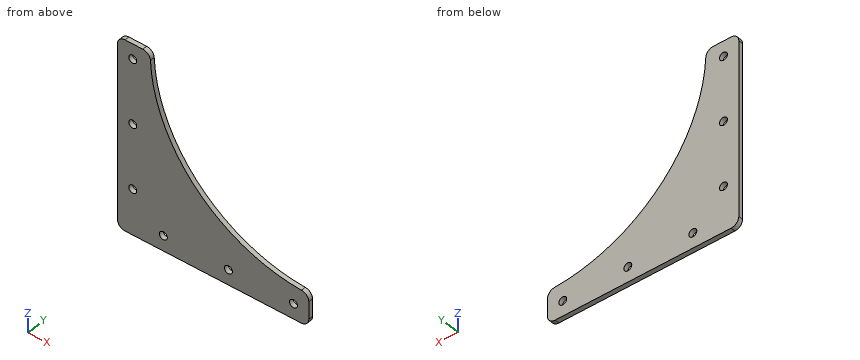
from build123d import *

# Parameters (mm, degrees)
F0_R     = 2.6
F1_DEPTH = 3


with BuildPart() as f1:
    # F0 (on Front) → F1 (new body)
    with BuildSketch(Plane.XZ):
        with BuildLine():
            Line((-57.5, -62.5), (57.5, -62.5))
            ThreePointArc((57.5, -62.5), (61.035534, -61.035534), (62.5, -57.5))
            Line((62.5, -57.5), (62.5, -45.930671))
            ThreePointArc((62.5, -45.930671), (61.116047, -42.477526), (57.730317, -40.935978))
            ThreePointArc((57.730317, -40.935978), (-10.718001, -10.718001), (-40.935978, 57.730317))
            ThreePointArc((-40.935978, 57.730317), (-42.477526, 61.116047), (-45.930671, 62.5))
            Line((-45.930671, 62.5), (-57.5, 62.5))
            ThreePointArc((-57.5, 62.5), (-61.035534, 61.035534), (-62.5, 57.5))
            Line((-62.5, 57.5), (-62.5, -57.5))
            ThreePointArc((-62.5, -57.5), (-61.035534, -61.035534), (-57.5, -62.5))
        make_face()
        with Locations((-32.5, -52.5)):
            Circle(F0_R, mode=Mode.SUBTRACT)
        with Locations((-52.5, -32.5)):
            Circle(F0_R, mode=Mode.SUBTRACT)
        with Locations((10, -52.5)):
            Circle(F0_R, mode=Mode.SUBTRACT)
        with Locations((52.5, -52.5)):
            Circle(F0_R, mode=Mode.SUBTRACT)
        with Locations((-52.5, 10)):
            Circle(F0_R, mode=Mode.SUBTRACT)
        with Locations((-52.5, 52.5)):
            Circle(F0_R, mode=Mode.SUBTRACT)
    extrude(amount=F1_DEPTH)


solid = f1.part
Geometry check sheet. Reference: the model listing, model coordinates, mm. Give positions to 0.01 mm unless a question says otherwise; leave off trailing zeros. Write each loop counter-clockwise with the first axis right and the second up, starting at its lowest first coordinate (ties: lowest second). Pieces come first, ordered by that corner, then holes. Notation, with made-up numbers: M 62.5,8.5 L 72.5,8.5 A22 cw 72.5,36.5 Z; hole C 84.5,36 d8. An arc over 180 degrees is marked long. Answer as CSV lines item,"result". Start each with the question number.
Q1. Section check B-B, the plane y = -2.05. Record the cut outline in (x, z).
Q2. Section check D-D, the plane z = 10. Record the cut outline in (x, y), then the cut area to 3 significant figures.
Q3. Go/stop test with a flat-tipped pin: pin 1 (1.5 mm diameter, centred on x = 5, y = -1.5, fed in from +Z). Record where the tip stops, or that it passes through.
Q4. Section check C-C, the plane x = 52.5. Record the cut outline in (y, z), then the cut area to 3 significant figures.
Q5. Material ranges on L1, parallel to Z at x = -52.5, y = -0.9; L2, parallel to X at y = -1.55, z = -54; L3, parallel to X at y = -1.6, z = -31.5, recorded low to high.
Q6. Section check A-A, the plane z = -52.5. Record the cut outline in (x, y), then the cut area to 3 significant figures.
Geometry says:
1,outline,"M -62.5,-57.5 A5 ccw -57.5,-62.5 L 57.5,-62.5 A5 ccw 62.5,-57.5 L 62.5,-45.93 A5 ccw 57.73,-40.94 A103.55 cw -40.94,57.73 A5 ccw -45.93,62.5 L -57.5,62.5 A5 ccw -62.5,57.5 Z; hole C -52.5,-32.5 d5.2; hole C -52.5,10 d5.2; hole C -52.5,52.5 d5.2; hole C -32.5,-52.5 d5.2; hole C 10,-52.5 d5.2; hole C 52.5,-52.5 d5.2"
2,outline,"M -62.5,-3 L -55.1,-3 L -55.1,0 L -62.5,0 Z; M -49.9,-3 L -26.75,-3 L -26.75,0 L -49.9,0 Z"
2,area,"91.7 mm^2"
3,pin 1,"z = -23.11"
4,outline,"M -3,-62.5 L 0,-62.5 L 0,-55.1 L -3,-55.1 Z; M -3,-49.9 L 0,-49.9 L 0,-40.56 L -3,-40.56 Z"
4,area,"50.2 mm^2"
5,L1,"-62.5 to -35.1, -29.9 to 7.4, 12.6 to 49.9, 55.1 to 62.5"
5,L2,"-62.5 to -34.62, -30.38 to 7.88, 12.12 to 50.38, 54.62 to 62.5"
5,L3,"-62.5 to -54.9, -50.1 to 19.07"
6,outline,"M -62.5,-3 L -35.1,-3 L -35.1,0 L -62.5,0 Z; M -29.9,-3 L 7.4,-3 L 7.4,0 L -29.9,0 Z; M 12.6,-3 L 49.9,-3 L 49.9,0 L 12.6,0 Z; M 55.1,-3 L 62.5,-3 L 62.5,0 L 55.1,0 Z"
6,area,"328 mm^2"
